```python
from build123d import *

# Parameters (mm, degrees)
SKETCH_2_W          = 88.9
SKETCH_2_H          = 3
EXTRUDE_1_DEPTH     = 88.9
SKETCH_4_R          = 1.5
SKETCH_4_W          = 2.88
SKETCH_4_H          = 9.6
SKETCH_4_W_2        = 9.6
SKETCH_4_H_2        = 2.88
CUT_EXTRUDE_1_DEPTH = 3
SKETCH_5_R          = 1.56
CUT_EXTRUDE_2_DEPTH = 3
SKETCH_7_R          = 2.495
CUT_EXTRUDE_3_DEPTH = 3
SKETCH_8_R          = 2.286
CUT_EXTRUDE_4_DEPTH = 3


with BuildPart() as part:
    # 스케치2 → 보스-돌출1 (new body)
    with BuildSketch(Plane.XY):
        Rectangle(SKETCH_2_W, SKETCH_2_H)
    extrude(amount=EXTRUDE_1_DEPTH)

    # 스케치4 → 컷-돌출1 (cut)
    with BuildSketch(Plane(origin=(0, 1.5, 0), x_dir=(1, 0, 0), z_dir=(0, 1, 0))):
        with Locations(Location((-41.275, -85.725, 0), (0, 0, 270))):
            Circle(SKETCH_4_R)
        with Locations(Location((-41.275, -3.175, 0), (0, 0, 270))):
            Circle(SKETCH_4_R)
        with Locations(Location((41.275, -3.175, 0), (0, 0, 270))):
            Circle(SKETCH_4_R)
        with Locations(Location((41.275, -85.725, 0), (0, 0, 270))):
            Circle(SKETCH_4_R)
        with Locations((-36.6, -69.85)):
            Rectangle(SKETCH_4_W, SKETCH_4_H)
        with Locations((-36.6, -19.05)):
            Rectangle(SKETCH_4_W, SKETCH_4_H)
        with Locations((-25.4, -7.85)):
            Rectangle(SKETCH_4_W_2, SKETCH_4_H_2)
        with Locations((36.6, -69.85)):
            Rectangle(SKETCH_4_W, SKETCH_4_H)
        with Locations((36.6, -19.05)):
            Rectangle(SKETCH_4_W, SKETCH_4_H)
        with Locations((25.4, -7.85)):
            Rectangle(SKETCH_4_W_2, SKETCH_4_H_2)
        with Locations((25.4, -81.05)):
            Rectangle(SKETCH_4_W_2, SKETCH_4_H_2)
        with Locations((-25.4, -81.05)):
            Rectangle(SKETCH_4_W_2, SKETCH_4_H_2)
    extrude(amount=-CUT_EXTRUDE_1_DEPTH, mode=Mode.SUBTRACT)

    # 스케치5 → 컷-돌출2 (cut)
    with BuildSketch(Plane(origin=(0, 1.5, 0), x_dir=(1, 0, 0), z_dir=(0, 1, 0))):
        with Locations(Location((-14.431818182, -30.018181818, 0), (0, 0, 270))):
            Circle(SKETCH_5_R)
        with Locations(Location((14.431818182, -30.018181818, 0), (0, 0, 270))):
            Circle(SKETCH_5_R)
        with Locations(Location((14.431818182, -58.881818182, 0), (0, 0, 270))):
            Circle(SKETCH_5_R)
        with Locations(Location((-14.431818182, -58.881818182, 0), (0, 0, 270))):
            Circle(SKETCH_5_R)
    extrude(amount=-CUT_EXTRUDE_2_DEPTH, mode=Mode.SUBTRACT)

    # 스케치7 → 컷-돌출3 (cut)
    with BuildSketch(Plane(origin=(0, 1.5, 0), x_dir=(1, 0, 0), z_dir=(0, 1, 0))):
        with Locations(Location((14.431818182, -30.018181818, 0), (0, 0, 270))):
            Circle(SKETCH_7_R)
        Polygon((6.401818182, -51.503445681), (2.941818182, -49.50581375), (2.941818182, -45.510549887), (6.401818182, -43.512917955), (9.861818182, -45.510549887), (9.861818182, -49.50581375), align=None)
        Polygon((4.40418625, -15.988181818), (2.406554319, -12.528181818), (4.40418625, -9.068181818), (8.399450113, -9.068181818), (10.397082045, -12.528181818), (8.399450113, -15.988181818), align=None)
    extrude(amount=-CUT_EXTRUDE_3_DEPTH, mode=Mode.SUBTRACT)

    # 스케치8 → 컷-돌출4 (cut)
    with BuildSketch(Plane(origin=(0, 1.5, 0), x_dir=(1, 0, 0), z_dir=(0, 1, 0))):
        with Locations(Location((0, -44.45, 0), (0, 0, 270))):
            Circle(SKETCH_8_R)
    extrude(amount=-CUT_EXTRUDE_4_DEPTH, mode=Mode.SUBTRACT)


solid = part.part
```
Part model, mm, in its own coordinate system. Round coordinates to 2 decimals unless told otherwise and drop trailing zeros. Loops run counter-clockwise (first coordinate to the right, second up) from the corner with the lowest first, then second, coordinate; pieces in that order, holes last.
Item 1: Drop a flat-ended pin along its axis: P1, Ø2.5, axis at x = 14.43, z = 58.88, coming from the +Y side. Give the stop position or say it passes through.
Item 2: Cut at D-D, the plane y = -0.7. State how many separate pieces and enclosed holes the cut face has, then the cut area to 3 significant figures.
Item 3: Drill centre lines: line 1 (X direction, y = 1.35, z = 17.5); line 2 (Z direction, x = -26, y = 1); line 3 (Z direction, x = -14.5, y = -1). Where is each one in solid material? Low to high.
Item 4: Cut at B-B, the plane x = 0. Give the cut face in (y, z), then the cut area to 3 significant figures.
Item 5: Cut at C-C, the plane z = 68. Give the cut face in (x, y), then the cut area to 3 significant figures.
Item 6: Cut at A-A, the plane x = 23. Give the cut face in (y, z).
A:
1. P1: passes through
2. separate pieces: 1
2. enclosed holes: 19
2. area: 7,510 mm2
3. line 1: x = -44.45 to -38.04, -35.16 to 35.16, 38.04 to 44.45
3. line 2: z = 0 to 6.41, 9.29 to 79.61, 82.49 to 88.9
3. line 3: z = 0 to 28.46, 31.58 to 57.32, 60.44 to 88.9
4. outline: (-1.5, 0) - (1.5, 0) - (1.5, 42.16) - (-1.5, 42.16) - close; (-1.5, 46.74) - (1.5, 46.74) - (1.5, 88.9) - (-1.5, 88.9) - close
4. area: 253 mm2
5. outline: (-44.45, -1.5) - (-38.04, -1.5) - (-38.04, 1.5) - (-44.45, 1.5) - close; (-35.16, -1.5) - (35.16, -1.5) - (35.16, 1.5) - (-35.16, 1.5) - close; (38.04, -1.5) - (44.45, -1.5) - (44.45, 1.5) - (38.04, 1.5) - close
5. area: 249 mm2
6. outline: (-1.5, 0) - (1.5, 0) - (1.5, 6.41) - (-1.5, 6.41) - close; (-1.5, 9.29) - (1.5, 9.29) - (1.5, 79.61) - (-1.5, 79.61) - close; (-1.5, 82.49) - (1.5, 82.49) - (1.5, 88.9) - (-1.5, 88.9) - close
